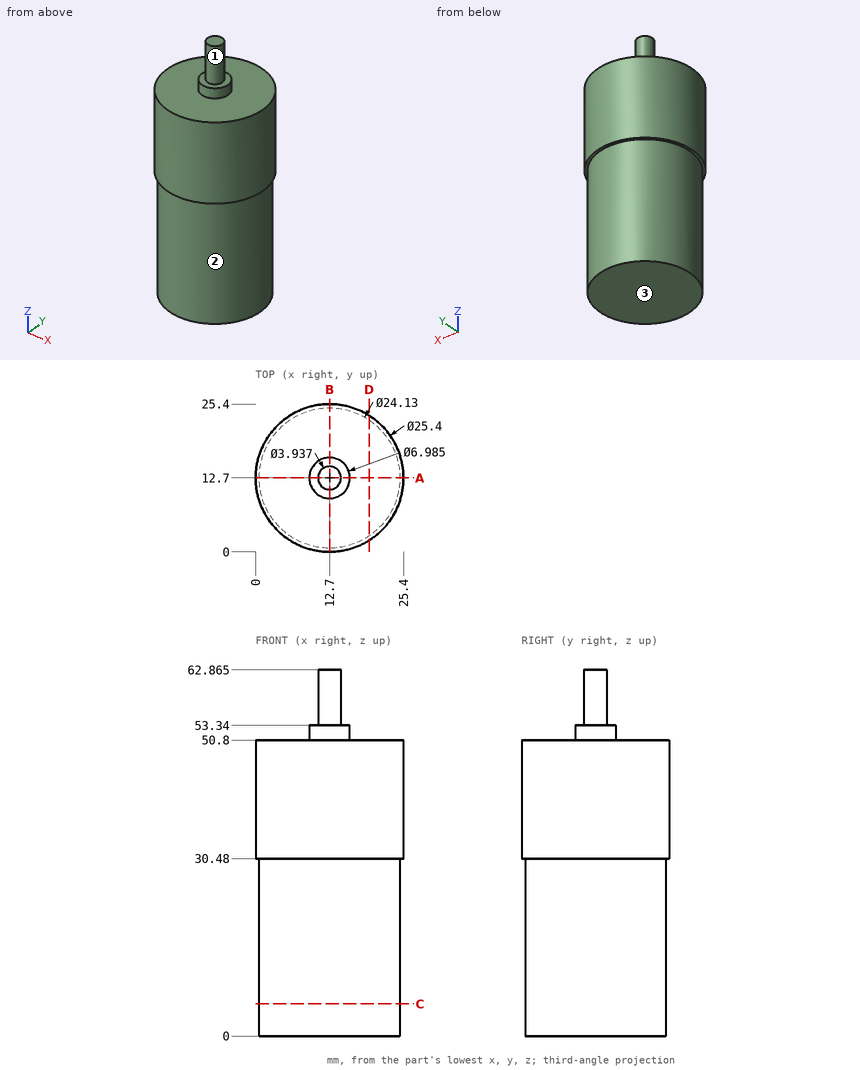
Input: dimensioned drawing with shaded views. Units: mm. Origin: part minimum x, y, z. A direction names the side the tool comes from. Give positions to 0.01 mm unless a question says otherwise; leave off trailing zeros. Order: outer loops, then holes, each group sorted by start corner. A loop starts at its lowest first (then second) coordinate and runs counter-clockwise, first axis right, second up.
(1) Section query D-D (x = 19.5). Return the cut outline in (y, z).
(2) Section query A-A (y = 12.7). Return the cut outline in (x, z) (1 decimal).
(3) Section query C-C (z = 5.5). Return the cut outline in (x, y) (3 decimals).
(4) Material intervals for line 1 along Z through (x, y) = (17.25, 14); line 2 along Z through (x, y) = (1.75, 7); line 3 along Y through (x, z) = (13.25, 23.5), sorted ascending.
(5) Contact query for flat-ended pins moving along their axis: P1, Ø2, axis at y = 13, z = 11.5, coming from the -X side (3 decimals); P2, Ø1.5, axis at x = 15.5, y = 22.5, coming from the +Z side; P3, Ø6, axis at x = 7.5, z = 40, coming from the +Y side. Output: stop coordinate, or through.
(6) Access query for the marked faces 1, 2 and 3. Directions: +Z, -Z, +X, -X, +Y, -Y. A direction counts if a zero-diameter tool reaches every point of the face in a straight line with its end or side. Return the directions, or none.
Outcome:
1. outline: (1.97, 30.48) - (2.73, 30.48) - (2.73, 0) - (22.67, 0) - (22.67, 30.48) - (23.43, 30.48) - (23.43, 50.8) - (1.97, 50.8) - close
2. outline: (0, 30.5) - (0.6, 30.5) - (0.6, 0) - (24.8, 0) - (24.8, 30.5) - (25.4, 30.5) - (25.4, 50.8) - (16.2, 50.8) - (16.2, 53.3) - (14.7, 53.3) - (14.7, 62.9) - (10.7, 62.9) - (10.7, 53.3) - (9.2, 53.3) - (9.2, 50.8) - (0, 50.8) - close
3. outline: circle Ø24.13 at (12.7, 12.7)
4. line 1: z = 0 to 50.8
4. line 2: z = 30.48 to 50.8
4. line 3: y = 0.65 to 24.75
5. P1: stops at x = 0.635
5. P2: stops at z = 50.8
5. P3: stops at y = 25.21
6. face 1: +Z
6. face 2: -Z
6. face 3: -Z, +X, -X, +Y, -Y
